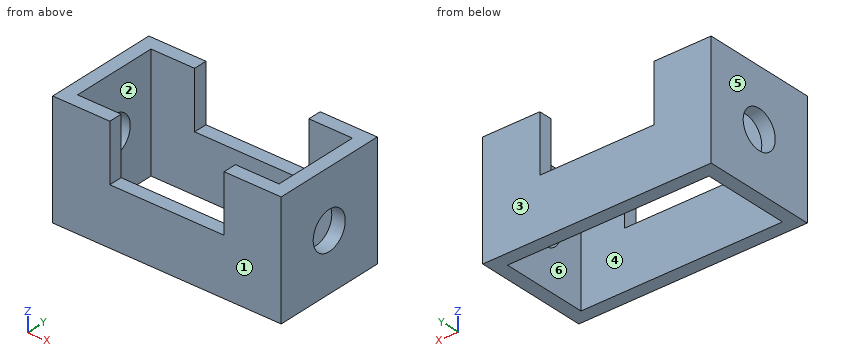
from build123d import *

# Parameters (mm, degrees)
F0_W     = 152.4
F0_H     = 76.2
F0_W_2   = 134.439488
F0_H_2   = 58.239488
F1_DEPTH = 76.2
F2_W     = 76.2
F2_H     = 38.1
F3_DEPTH = 25.4
F4_W     = 76.2
F4_H     = 38.1
F5_DEPTH = 25.4
F6_R     = 12.7
F7_DEPTH = 51.562
F8_R     = 12.7
F9_DEPTH = 25.4


with BuildPart() as f1:
    # F0 (on Top) → F1 (new body)
    with BuildSketch(Plane.XY):
        with Locations((-3.510571, 16.603382)):
            Rectangle(F0_W, F0_H)
        with Locations((-3.510571, 16.603382)):
            Rectangle(F0_W_2, F0_H_2, mode=Mode.SUBTRACT)
    extrude(amount=F1_DEPTH)

    # F2 (on face) → F3 (cut)
    with BuildSketch(Plane.XZ.offset(21.496618)):
        with Locations((-3.510571, 57.15)):
            Rectangle(F2_W, F2_H)
    extrude(amount=-F3_DEPTH, mode=Mode.SUBTRACT)

    # F4 (on face) → F5 (cut)
    with BuildSketch(Plane(origin=(0, 54.703382, 0), x_dir=(-1, 0, 0), z_dir=(0, 1, 0))):
        with Locations((3.510571, 57.15)):
            Rectangle(F4_W, F4_H)
    extrude(amount=-F5_DEPTH, mode=Mode.SUBTRACT)

    # F6 (on face) → F7 (cut)
    with BuildSketch(Plane(origin=(-79.710571, 0, 0), x_dir=(0, -1, 0), z_dir=(-1, 0, 0))):
        with Locations((-16.603382, 38.1)):
            Circle(F6_R)
    extrude(amount=-F7_DEPTH, mode=Mode.SUBTRACT)

    # F8 (on face) → F9 (cut)
    with BuildSketch(Plane.YZ.offset(72.689429)):
        with Locations((16.603382, 38.1)):
            Circle(F8_R)
    extrude(amount=-F9_DEPTH, mode=Mode.SUBTRACT)


solid = f1.part
Geometry: final body of the model. Coordinates: model frame, mm. Face numbers are marked on the shaded views. A direction names the side the tool comes from. Give positions to 0.01 mm unless a question says otherwise; leave off trailing zeros. Write each loop counter-clockwise with the first axis right and the second up, starting at its lowest first coordinate (ties: lowest second). Pieces come first, ordered by that corner, then holes. Notation, with made-up numbers: M -36.75,51.25 L -29.75,51.25 A18 cw -29.75,56.25 Z; hole C -9,77.5 d11. An arc over 180 degrees is marked long. Answer in a Markdown table with one row per item. Add a question column.
(1) Section C-C on y = -1. Return loops of the section in (x, z).
(2) Section B-B on z = 69. Return loops of the section in (x, y), and give its area (3 significant figures).
(3) Section A-A on x = 42. Return loops of the section in (y, z).
(4) First-contact query: pin 1 (7 mm diameter, centred on x = -11.5, y = -19, fed in from +Z). Flat tip, straight axial feed; report the tip coordinate or a pass-through.
(5) Mould query, pull axis Y, two halves, no side actions, for the marked faces 3, 4, 5 and 6. Classes: +Y half, -Y half, draft (parallel to the pull), parting line (faces both ways), or undercut.
(6) Reachability of the marked faces 1 and 2 from +Z, -Z, +X, -X, +Y, -Y: full face, straight path, thin tool, end or side. Return the list, or none.
(7) Section D-D on y = -14.5. Return loops of the section in (x, z).
(8) Ray query, line 1 (X direction, y = -6.5, z = 36.5); line 2 (Y direction, x = -9, z = 15); line 3 (X direction, y = 47.5, z = 48). Return the intervals inside material, ascending.
Result set:
| question | item | result |
|---|---|---|
| 1 | outline | M -79.71,0 L -70.73,0 L -70.73,76.2 L -79.71,76.2 Z; M 63.71,0 L 72.69,0 L 72.69,76.2 L 63.71,76.2 Z |
| 2 | outline | M -79.71,-21.5 L -41.61,-21.5 L -41.61,-12.52 L -70.73,-12.52 L -70.73,45.72 L -41.61,45.72 L -41.61,54.7 L -79.71,54.7 Z; M 34.59,-21.5 L 72.69,-21.5 L 72.69,54.7 L 34.59,54.7 L 34.59,45.72 L 63.71,45.72 L 63.71,-12.52 L 34.59,-12.52 Z |
| 2 | area | 2,410 mm^2 |
| 3 | outline | M -21.5,0 L -12.52,0 L -12.52,76.2 L -21.5,76.2 Z; M 45.72,0 L 54.7,0 L 54.7,76.2 L 45.72,76.2 Z |
| 4 | pin 1 | stops at z = 38.1 |
| 5 | face 3 | +Y half |
| 5 | face 4 | undercut |
| 5 | face 5 | draft |
| 5 | face 6 | undercut |
| 6 | face 1 | +Z, -Z, +X, -X, -Y |
| 6 | face 2 | +Z, -Z |
| 7 | outline | M -79.71,0 L 72.69,0 L 72.69,76.2 L 34.59,76.2 L 34.59,38.1 L -41.61,38.1 L -41.61,76.2 L -79.71,76.2 Z |
| 8 | line 1 | x = -79.71 to -70.73, 63.71 to 72.69 |
| 8 | line 2 | y = -21.5 to -12.52, 45.72 to 54.7 |
| 8 | line 3 | x = -79.71 to -41.61, 34.59 to 72.69 |
